The model under review builds one solid part; all positions refer to its coordinate system, in mm. A direction names the side the tool comes from. Coordinates: 2 decimals unless noted, no trailing zeros. Loops run counter-clockwise (first coordinate to the right, second up) from the corner with the lowest first, then second, coordinate; pieces in that order, holes last. Notation, with made-up numbers: (32.5, 76) - (91.5, 76) arc R28 ccw to (91.5, 102) - close; hole circle Ø5 at (54, -16). An arc over 180 degrees is marked (long way). Answer in a Markdown table with one row per item. Add a question column.
(1) Mouldability with a two-part tool opening along Z and no side actions: class faces 1 (the cylindrical face through (12.204, -9.569, 146.018)), 2 (the flat face through (13, -9, 165.1)), 3 (the flat face through (13, -12.7, 109)), 4 (the flat face through (13, -10, 50.8)) as +Z half, -Z half, draft (parallel to the pull), parting line (faces both ways), or undercut.
(2) For P1, Ø7, axis at x = 12.7, z = 142.24, coming from the +Y side; P2, Ø12.5, axis at x = 14.5, z = 147, coming from the +Y side; P3, Ø5, axis at x = 17.5, y = -3.5, coming from the +Z side; P4, Ø12.5, axis at x = 11.5, z = 25.5, coming from the -Y side, all flat-tipped, find the tip position at first contact; note any pin that passes through.
(3) Machinability: for faces 5 (the flat face through (13, -6.35, 26)), 6 (the flat face through (13, -3, 0)), 7 (the flat face through (13, -6.35, 134)), which of the approach directions +Z, -Z, +X, -X, +Y, -Y give a long, thin tool a straight path to every point of the face, cutting with its end or side? Answer none if there is none.
(4) We need section D-D on z = 124. Write out the cut boundary in (x, y).
(5) We need section C-C on x = 22.25. Write out the cut boundary in (y, z), plus the area to 3 significant figures.
(6) We need section A-A on x = 12.7. Write out the cut boundary in (y, z).
(7) For line 1 along Z through (x, y) = (12.7, -11); line 2 along X through (y, z) = (-8.25, 142.24); line 3 along Z through (x, y) = (13.5, -5), list the stretches that pass through material, from the lowest coordinate up.
(8) We need section B-B on y = -10.25. Write out the cut boundary in (x, z).
from build123d import *

# Parameters (mm, degrees)
F0_W     = 25.4
F0_H     = 165.1
F1_DEPTH = 12.7
F2_W     = 25.4
F2_H     = 50.8
F3_DEPTH = 6.35
F4_DEPTH = 6.35
F5_W     = 25.4
F5_H     = 50.8
F6_DEPTH = 6.35
F7_R     = 3.81
F8_DEPTH = 25.4


with BuildPart() as f1:
    # F0 (on Front) → F1 (new body)
    with BuildSketch(Plane.XZ):
        with Locations((12.7, 82.55)):
            Rectangle(F0_W, F0_H)
    extrude(amount=F1_DEPTH)

    # F2 (on face) → F3 (join)
    with BuildSketch(Plane.XZ.offset(12.7)):
        with Locations((12.7, 25.4)):
            Rectangle(F2_W, F2_H)
    extrude(amount=-F3_DEPTH)

    # F2 (on face) → F4 (cut)
    with BuildSketch(Plane.XZ.offset(12.7)):
        with Locations((12.7, 25.4)):
            Rectangle(F2_W, F2_H)
    extrude(amount=-F4_DEPTH, mode=Mode.SUBTRACT)

    # F5 (on face) → F6 (cut)
    with BuildSketch(Plane(origin=(0, 0, 0), x_dir=(-1, 0, 0), z_dir=(0, 1, 0))):
        with Locations((-12.7, 139.7)):
            Rectangle(F5_W, F5_H)
    extrude(amount=-F6_DEPTH, mode=Mode.SUBTRACT)

    # F7 (on face) → F8 (cut)
    with BuildSketch(Plane.XZ.offset(12.7)):
        with Locations((12.7, 142.24)):
            Circle(F7_R)
    extrude(amount=-F8_DEPTH, mode=Mode.SUBTRACT)


solid = f1.part
Outcome:
| question | item | result |
|---|---|---|
| 1 | face 1 | undercut |
| 1 | face 2 | +Z half |
| 1 | face 3 | draft |
| 1 | face 4 | -Z half |
| 2 | P1 | through |
| 2 | P2 | y = -6.35 |
| 2 | P3 | z = 114.3 |
| 2 | P4 | y = -6.35 |
| 3 | face 5 | -Z, +X, -X, -Y |
| 3 | face 6 | -Z, +X, -X, +Y, -Y |
| 3 | face 7 | +Z, +X, -X, +Y |
| 4 | outline | (0, -12.7) - (25.4, -12.7) - (25.4, -6.35) - (0, -6.35) - close |
| 5 | outline | (-12.7, 50.8) - (-6.35, 50.8) - (-6.35, 0) - (0, 0) - (0, 114.3) - (-6.35, 114.3) - (-6.35, 165.1) - (-12.7, 165.1) - close |
| 5 | area | 1,450 mm² |
| 6 | outline | (-12.7, 50.8) - (-6.35, 50.8) - (-6.35, 0) - (0, 0) - (0, 114.3) - (-6.35, 114.3) - (-6.35, 138.43) - (-12.7, 138.43) - close; (-12.7, 146.05) - (-6.35, 146.05) - (-6.35, 165.1) - (-12.7, 165.1) - close |
| 7 | line 1 | 50.8 to 138.43, 146.05 to 165.1 |
| 7 | line 2 | 0 to 8.89, 16.51 to 25.4 |
| 7 | line 3 | 0 to 114.3 |
| 8 | outline | (0, 50.8) - (25.4, 50.8) - (25.4, 165.1) - (0, 165.1) - close; hole circle Ø7.62 at (12.7, 142.24) |
